For this review, use the dimensioned drawing (mm, ordinates from the lowest corner) and the shaded views. Coordinates: 2 decimals unless noted, no trailing zeros. Loops run counter-clockwise (first coordinate to the right, second up) from the corner with the lowest first, then second, coordinate; pieces in that order, holes last. Notation, with made-up numbers: (35.5, 83) - (41.5, 83) arc R21 cw to (41.5, 116) - close; hole circle Ø8 at (-38, 87.25). An arc over 180 degrees is marked (long way). Answer in a Markdown table with one row per item. Add a question column.
(1) For line 1 along X through (y, z) = (2.4, 60); line 2 along X through (y, z) = (2.4, 57.5); line 3 along X through (y, z) = (3.05, 9.5), list the stretches that pass through material, from the lowest coordinate up.
(2) We need section A-A on z = 60. Write out the cut boundary in (x, y).
(3) We need section B-B on x = 85. Write out the cut boundary in (y, z), plus the area to 3 significant figures.
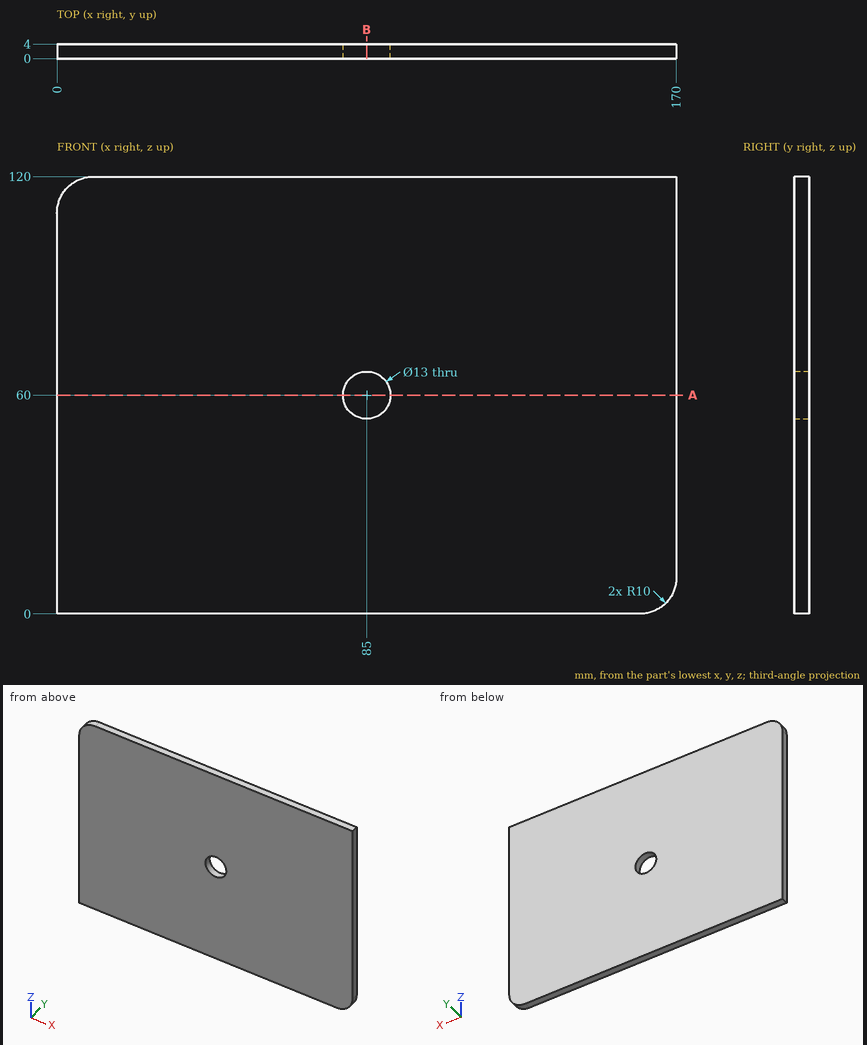
Outcome:
| question | item | result |
|---|---|---|
| 1 | line 1 | 0 to 78.5, 91.5 to 170 |
| 1 | line 2 | 0 to 79, 91 to 170 |
| 1 | line 3 | 0 to 169.99 |
| 2 | outline | (0, 0) - (78.5, 0) - (78.5, 4) - (0, 4) - close; (91.5, 0) - (170, 0) - (170, 4) - (91.5, 4) - close |
| 3 | outline | (0, 0) - (4, 0) - (4, 53.5) - (0, 53.5) - close; (0, 66.5) - (4, 66.5) - (4, 120) - (0, 120) - close |
| 3 | area | 428 mm² |
